Read the model definition and answer for the solid it produces. Units are mm, in the model's axes. Give positions to 0.01 mm unless a question says otherwise; leave off trailing zeros. Order: outer loops, then holes, each group sorted by start corner. A loop starts at its lowest first (then second) coordinate and runs counter-clockwise, first axis right, second up.
Item 1: Given pin 1 Ø2.5 at (x, y) = (-0.5, 1.5) entering from +Z; pin 2 Ø1 at (x, z) = (2.5, 64) entering from +Y; pin 3 Ø1 at (x, z) = (0, 22) entering from +Y; pin 4 Ø6 at (y, z) = (-3, 49) entering from +X, each flat-ended and moving along its own axis, determine where each tip first touches the part or whether it passes through.
Item 2: Find the intervals of material crossed by line 1 along Z through (x, y) = (-4.25, 0.75); line 2 along Y through (x, z) = (0, -0.5); line 3 along X through (y, z) = (0.25, 18.5), in increasing order.
Item 3: A cutting plane is placed at D-D (y = 3.5). Write down the section's boundary in (x, z).
Item 4: A cutting plane is placed at A-A (y = 0). Write down the section's boundary in (x, z), plus the area to 3 significant figures.
Item 5: A cutting plane is placed at C-C (z = 9). Write down the section's boundary in (x, y).
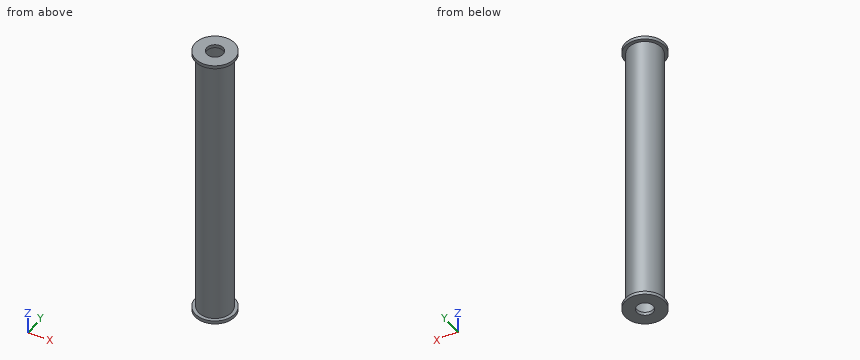
from build123d import *

# Parameters (mm, degrees)
SKETCH1_R           = 5
SKETCH1_R_2         = 4.5
BOSS_EXTRUDE1_DEPTH = 84.88
SKETCH2_R           = 6
SKETCH2_R_2         = 2.5
BOSS_EXTRUDE2_DEPTH = 1
SKETCH3_R           = 6
SKETCH3_R_2         = 2.5
BOSS_EXTRUDE3_DEPTH = 1


with BuildPart() as part:
    # Sketch1 → Boss-Extrude1 (new body)
    with BuildSketch(Plane.XY):
        Circle(SKETCH1_R)
        Circle(SKETCH1_R_2, mode=Mode.SUBTRACT)
    extrude(amount=BOSS_EXTRUDE1_DEPTH)

    # Sketch2 → Boss-Extrude2 (add)
    with BuildSketch(Plane(origin=(0, 0, 0), x_dir=(-1, 0, 0), z_dir=(0, 0, -1))):
        Circle(SKETCH2_R)
        Circle(SKETCH2_R_2, mode=Mode.SUBTRACT)
    extrude(amount=BOSS_EXTRUDE2_DEPTH)

    # Sketch3 → Boss-Extrude3 (add)
    with BuildSketch(Plane.XY.offset(84.88)):
        Circle(SKETCH3_R)
        Circle(SKETCH3_R_2, mode=Mode.SUBTRACT)
    extrude(amount=BOSS_EXTRUDE3_DEPTH)


solid = part.part
Response values:
1. pin 1: stops at z = 85.88
1. pin 2: stops at y = 4.58
1. pin 3: stops at y = 5
1. pin 4: stops at x = 5
2. line 1: z = -1 to 0, 84.88 to 85.88
2. line 2: y = -6 to -2.5, 2.5 to 6
2. line 3: x = -4.99 to -4.49, 4.49 to 4.99
3. outline: (-4.87, -1) - (4.87, -1) - (4.87, 0) - (3.57, 0) - (3.57, 84.88) - (4.87, 84.88) - (4.87, 85.88) - (-4.87, 85.88) - (-4.87, 84.88) - (-3.57, 84.88) - (-3.57, 0) - (-4.87, 0) - close; hole (-2.83, 0) - (2.83, 0) - (2.83, 84.88) - (-2.83, 84.88) - close
4. outline: (-6, -1) - (-2.5, -1) - (-2.5, 0) - (-4.5, 0) - (-4.5, 84.88) - (-2.5, 84.88) - (-2.5, 85.88) - (-6, 85.88) - (-6, 84.88) - (-5, 84.88) - (-5, 0) - (-6, 0) - close; (2.5, -1) - (6, -1) - (6, 0) - (5, 0) - (5, 84.88) - (6, 84.88) - (6, 85.88) - (2.5, 85.88) - (2.5, 84.88) - (4.5, 84.88) - (4.5, 0) - (2.5, 0) - close
4. area: 98.9 mm2
5. outline: circle Ø10 at (0, 0); hole circle Ø9 at (0, 0)
